Design review of the part built by this model. Coordinates are the model's own, in mm. A direction names the side the tool comes from. Coordinates: 2 decimals unless noted, no trailing zeros. Write each loop counter-clockwise with the first axis right and the second up, starting at its lowest first coordinate (ties: lowest second). Pieces come first, ordered by that corner, then holes. Notation, with made-up numbers: M -22,10.25 L 14,10.25 A12 cw 14,28.25 Z; hole C 88.25,-34.75 d10. An arc over 180 degrees is marked long. Write item = value, one per line.
```python
from build123d import *

# Parameters (mm, degrees)
SKETCH_1_W          = 130
SKETCH_1_H          = 100
SKETCH_1_W_2        = 105
SKETCH_1_H_2        = 75
EXTRUDE_1_DEPTH     = 3
SKETCH_2_W          = 111
SKETCH_2_H          = 81
SKETCH_2_W_2        = 105
SKETCH_2_H_2        = 75
EXTRUDE_2_DEPTH     = 73.5
FILLET_1_R          = 1.5
SKETCH_4_R          = 2.5
CUT_EXTRUDE_2_DEPTH = 113.5
CUT_EXTRUDE_4_DEPTH = 73.5
SKETCH_7_W          = 105
SKETCH_7_H          = 75
EXTRUDE_3_DEPTH     = 2.5


with BuildPart() as part:
    # 草图1 → 凸台-拉伸1 (new body)
    with BuildSketch(Plane.XY):
        Rectangle(SKETCH_1_W, SKETCH_1_H)
        Rectangle(SKETCH_1_W_2, SKETCH_1_H_2, mode=Mode.SUBTRACT)
    extrude(amount=EXTRUDE_1_DEPTH)

    # 草图2 → 凸台-拉伸2 (add)
    with BuildSketch(Plane.XY.offset(3)):
        Rectangle(SKETCH_2_W, SKETCH_2_H)
        Rectangle(SKETCH_2_W_2, SKETCH_2_H_2, mode=Mode.SUBTRACT)
    extrude(amount=EXTRUDE_2_DEPTH)

    # 圆角1
    fillet_1_edges = [part.edges().sort_by_distance(p)[0] for p in [
        (55.5, 0, 3),
        (0, 40.5, 3),
        (-55.5, 0, 3),
        (0, -40.5, 3),
    ]]
    fillet(fillet_1_edges, radius=FILLET_1_R)

    # 草图4 → 切除-拉伸2 (cut)
    with BuildSketch(Plane.XY.offset(3)):
        with Locations((-60.5, 45.5)):
            Circle(SKETCH_4_R)
        with Locations((60.5, 45.5)):
            Circle(SKETCH_4_R)
        with Locations((60.5, -45.5)):
            Circle(SKETCH_4_R)
        with Locations((-60.5, -45.5)):
            Circle(SKETCH_4_R)
    extrude(amount=-CUT_EXTRUDE_2_DEPTH, mode=Mode.SUBTRACT)

    # 草图6 → 切除-拉伸4 (cut)
    with BuildSketch(Plane.ZY.offset(55.5)):
        Polygon((25, 0), (47.5, -12.990381057), (47.5, 12.990381057), align=None)
    extrude(amount=-CUT_EXTRUDE_4_DEPTH, mode=Mode.SUBTRACT)

    # 草图7 → 凸台-拉伸3 (add)
    with BuildSketch(Plane.XY.offset(76.5)):
        Rectangle(SKETCH_7_W, SKETCH_7_H)
    extrude(amount=-EXTRUDE_3_DEPTH)


solid = part.part
```
Q1. Consider section C-C, the plane z = 68. State the section outline as (x, y) points, and give its area (3 significant figures).
Check result:
outline = M -55.5,-40.5 L 55.5,-40.5 L 55.5,40.5 L -55.5,40.5 Z; hole M -52.5,-37.5 L 52.5,-37.5 L 52.5,37.5 L -52.5,37.5 Z
area = 1,120 mm²
Q2. The part is to be moulded in two halves that separate along X. For faces 6 (the flat face through (-1, 37.5, 36)), 7 (the flat face through (-1, 1, 76.5)), 8 (the flat face through (55.5, -1, 40)), say which applies: +X half, -X half, draft (parallel to the pull), parting line (faces both ways), or undercut.
Check result:
face_6 = undercut
face_7 = draft
face_8 = +X half
Q3. Consider section B-B, the plane y = -45.5. State the section outline as (x, z) points.
Check result:
outline = M -65,0 L -63,0 L -63,3 L -65,3 Z; M -58,0 L 58,0 L 58,3 L -58,3 Z; M 63,0 L 65,0 L 65,3 L 63,3 Z
Q4. Consider section D-D, the plane x = 30. State the section outline as (y, z) points.
Check result:
outline = M -50,0 L -37.5,0 L -37.5,74 L 37.5,74 L 37.5,0 L 50,0 L 50,3 L 42,3 A1.5 cw 40.5,4.5 L 40.5,76.5 L -40.5,76.5 L -40.5,4.5 A1.5 cw -42,3 L -50,3 Z
Q5. For P1, Ø22.5, axis at x = -5.5, y = -15, coming from the -Z side; P2, Ø21.5, axis at y = 15.5, z = 55, coming from the -X side; P3, Ø4.5, axis at x = 60.5, y = 45.5, coming from the -Z side; P4, Ø12, axis at x = -23.5, z = 12, coming from the +Y side, all flat-tipped, find the tip position at first contact; note any pin that passes through.
Check result:
P1 = 74
P2 = -55.5
P3 = through
P4 = 40.5
Q6. Machinability: for faces 1 (the flat face through (52.5, -1, 36)), 2 (the flat face through (-54.021, -6.404, 36.092)), 3 (the flat face through (-1, 40.5, 40)), 4 (the flat face through (-55.5, -1, 48)), 5 (the flat face through (-1, -40.5, 40)), which of the approach directions +Z, -Z, +X, -X, +Y, -Y give a long, thin tool a straight path to every point of the face, cutting with its end or side? Answer none if there is none.
Check result:
face_1 = -Z
face_2 = -X
face_3 = +Z, +X, -X, +Y
face_4 = +Z, -X, +Y, -Y
face_5 = +Z, +X, -X, -Y
Q7. Wall thickness on line 1 (Y direction, x = -6, z = 61.5); line 2 (Y direction, x = 60.5, z = 1.15); line 3 (X direction, y = 34, z = 40): over which ranges is each line inside the solid? List them lowest first.
Check result:
line_1 = -40.5 to -37.5, 37.5 to 40.5
line_2 = -50 to -48, -43 to 43, 48 to 50
line_3 = -55.5 to -52.5, 52.5 to 55.5
Q8. Consider section A-A, the plane x = 60.5. State the section outline as (y, z) points.
Check result:
outline = M -50,0 L -48,0 L -48,3 L -50,3 Z; M -43,0 L 43,0 L 43,3 L -43,3 Z; M 48,0 L 50,0 L 50,3 L 48,3 Z
